The listing builds one solid part. Answer for the finished solid, in the listing's coordinates (mm). Coordinates: 2 decimals unless noted, no trailing zeros. Loops run counter-clockwise (first coordinate to the right, second up) from the corner with the lowest first, then second, coordinate; pieces in that order, holes last. Notation, with made-up numbers: M -29.75,76 L -4.75,76 A21 ccw -4.75,108 Z; hole C -1.5,48.25 d3. An arc over 180 degrees is marked long. Return JSON: item names as keys, results as strings. Group by question number.
1. Straight lines are drawn through the part: L1, parallel to X at y = 1, z = 4; L2, parallel to X at y = 16.5, z = 19; L3, parallel to Y at x = 0, z = 16. For each, find the intervals that lie inside material, in ascending order. Write a range as from..to.
2. Section A-A (z = 24.5) is taken. Write down the section's boundary in (x, y).
3. The mould has two halves that part along Y. Classify faces 1 (the face through (28.14, 8.86, 19.27)), 2 (the face through (-7.211, -32.475, 21.254)), 3 (the face through (-11.35, -27.43, 0)): pulls with the +Y half, pulls with the -Y half, needs draft (parallel to the pull), parting line crosses it, or undercut.
4. Section B-B (z = 8) is taken. Write down the section's boundary in (x, y).
5. Given P1, Ø5, axis at x = -25.5, y = -1, coming from the +Z side; P2, Ø10, axis at x = 23, z = 17, coming from the -Y side; P3, Ø10, axis at x = -13, z = 11, coming from the +Y side; P4, Ø10, axis at y = 0, z = 14, coming from the +X side, each flat-ended and moving along its own axis, determine where each tip first touches the part or whether it passes through.
```python
from build123d import *

# Parameters (mm, degrees)
F0_W     = 4
F0_H     = 40
F3_SIZE2 = 39.99999
F3_SIZE  = 0.49999
F4_R     = 2


# Not quite as in the source:
# - a fillet or chamfer is up to 0.001 mm smaller than in the source, because OpenCascade refuses the exact size


with BuildPart() as f2:
    # F0 (on Front) → F2 (revolve)
    with BuildSketch(Plane.XZ):
        with Locations((31.5, 20)):
            Rectangle(F0_W, F0_H)
    revolve(axis=Axis((0, 0, 14.9673912674), (0, 0, 1)))

    # F3 (size 0.5 and 40 in the source; OpenCascade refuses exactly that, so slightly less here)
    f3_edges = [f2.edges().sort_by_distance(p)[0] for p in [
        (-33.5, 0, 0),
    ]]
    chamfer(f3_edges, length=F3_SIZE, length2=F3_SIZE2)

    # F4
    f4_edges = [f2.edges().sort_by_distance(p)[0] for p in [
        (-29.5, 0, 40),
        (-33.00001, 0, 0),
    ]]
    fillet(f4_edges, radius=F4_R)


solid = f2.part
```
Worked out:
{
 "1": {"L1": "-33.03..-29.48, 29.48..33.03", "L2": "-28.85..-24.45, 24.45..28.85", "L3": "-33.2..-29.5, 29.5..33.2"},
 "2": {"outline": "C 0,0 d66.61; hole C 0,0 d59"},
 "3": {"face 1": "undercut", "face 2": "parting line crosses it", "face 3": "needs draft"},
 "4": {"outline": "C 0,0 d66.2; hole C 0,0 d59"},
 "5": {"P1": "through", "P2": "y = -27.91", "P3": "y = 32.16", "P4": "x = 33.24"}
}
